Autodesk Inventor part; units mm, degrees
ref_plane "YZ Plane" through (0, 0, 0) normal (1, 0, 0) x (0, 1, 0)
ref_plane "XZ Plane" through (0, 0, 0) normal (0, 1, 0) x (-1, 0, 0)
ref_plane "XY Plane" through (0, 0, 0) normal (0, 0, 1) x (1, 0, 0)
sketch "Náčrt1" plane through (0, 0, 0) normal (1, 0, 0) x (0, 1, 0)
  line L0 (0, 0) -> (0, -50)
  line L1 (0, -50) -> (80, -50)
  line L2 (80, -50) -> (80, 0)
  line L3 (80, 0) -> (0, 0)
  dimension "d0" = 50
  dimension "d1" = 80
  dimension "d2" = 50
extrude "Vysunutí1" add sketch "Náčrt1" along normal blind 50
sketch "Náčrt2" plane through (50, 0, 0) normal (1, 0, 0) x (0, 0, -1)
  line L0 (0, 0) -> (20, 0)
  line L1 (0, 0) -> (50, 0)
  line L2 (20, 0) -> (20, 15)
  line L3 (20, 15) -> (0, 15)
  line L4 (0, 80) -> (0, 0)
  line L5 (0, 0) -> (0, 15)
  line L6 (0, 80) -> (10, 80)
  line L7 (50, 80) -> (0, 80)
  line L8 (10, 80) -> (10, 65)
  line L9 (10, 65) -> (0, 65)
  line L10 (0, 80) -> (0, 65)
  dimension "d5" = 20
  dimension "d6" = 15
  dimension "d7" = 10
  dimension "d8" = 15
extrude "Vysunutí2" cut sketch "Náčrt2" against normal blind 50
sketch "Náčrt3" plane through (50, 0, 0) normal (1, 0, 0) x (0, 0, -1)
  line L0 (20, 0) -> (50, 0)
  line L1 (50, 0) -> (30, 0)
  line L2 (30, 0) -> (30, 80)
  line L3 (50, 80) -> (10, 80)
  line L4 (10, 80) -> (10, 65)
  line L5 (30, 80) -> (10, 80)
  line L6 (10, 80) -> (10, 65)
  line L7 (10, 65) -> (0, 65)
  line L8 (10, 65) -> (0, 65)
  line L9 (0, 15) -> (20, 15)
  line L10 (0, 65) -> (0, 15)
  line L11 (0, 15) -> (20, 15)
  line L12 (20, 15) -> (20, 0)
  line L13 (20, 15) -> (20, 0)
  line L14 (20, 0) -> (30, 0)
  point P0 (0, 0)
  dimension "d11" = 20
extrude "Vysunutí3" cut sketch "Náčrt3" against normal blind 20
properties part number "Martin-Probst-26673_obrazek_1"
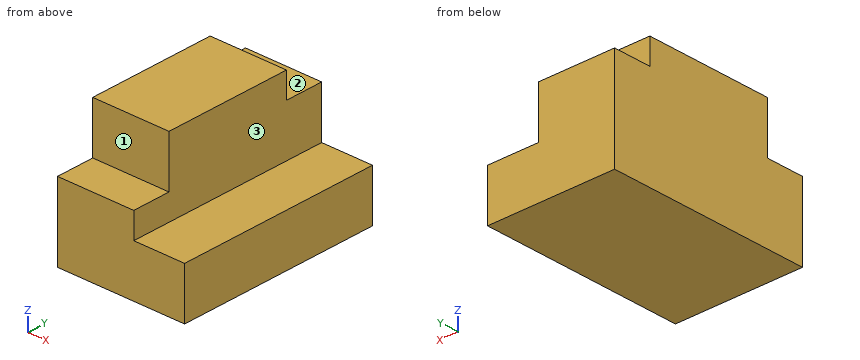
For this review, take the finished solid that the model builds, in its own axes (mm). Face numbers are marked on the shaded views. A direction names the side the tool comes from. Give positions to 0.01 mm unless a question says otherwise; leave off trailing zeros. Order: outer loops, then holes, each group sorted by start corner. A loop starts at its lowest first (then second) coordinate and runs counter-clockwise, first axis right, second up. Notation, with made-up numbers: (2.5, 15.5) - (57.5, 15.5) arc R18 ccw to (57.5, 38.5) - close; hole circle Ø10 at (20.25, 56). An arc over 180 degrees is marked (long way). Answer as a JSON object with one key per item and string values. Group by question number.
Item 1: Take a section at C-C on z = -28. Give the boundary of the cut face in (x, y).
Item 2: Take a section at B-B on x = 11.5. Give the boundary of the cut face in (y, z).
Item 3: Machinability: for the marked faces 1, 2 and 3, which of the approach directions +Z, -Z, +X, -X, +Y, -Y give a long, thin tool a straight path to every point of the face, cutting with its end or side? Answer none if there is none.
Item 4: Take a section at A-A on y = 52. Give the boundary of the cut face in (x, z), and give its area (3 significant figures).
Item 5: Clearance check with flat-ended pins moving along their axes: pin 1 Ø12 at (y, z) = (16, -19) entering from -X; pin 2 Ø4.5 at (x, y) = (17.5, 10) entering from +Z; pin 3 Ø10 at (x, y) = (37, 58.5) entering from +Z; pin 4 Ø10 at (x, z) = (11.5, -13) entering from -Y. State where each tip first meets the part, or that it passes through.
Item 6: Take a section at D-D on y = 14. Give the boundary of the cut face in (x, z).
Item 7: Wall thickness on line 1 along X through (y, z) = (39.5, -10); line 2 along Z through (x, y) = (35, 16); line 3 along Z through (x, y) = (21, 5): over which ranges is each line inside the solid? List them lowest first.
Reported:
{
 "1": {"outline": "(0, 0) - (30, 0) - (30, 80) - (0, 80) - close"},
 "2": {"outline": "(0, -50) - (80, -50) - (80, -10) - (65, -10) - (65, 0) - (15, 0) - (15, -20) - (0, -20) - close"},
 "3": {"face 1": "+Z, +X, -X, -Y", "face 2": "+Z, +X, -X, +Y", "face 3": "+Z, +X, +Y, -Y"},
 "4": {"outline": "(0, -50) - (50, -50) - (50, -30) - (30, -30) - (30, 0) - (0, 0) - close", "area": "1,900 mm^2"},
 "5": {"pin 1": "x = 0", "pin 2": "z = -20", "pin 3": "z = -30", "pin 4": "y = 15"},
 "6": {"outline": "(0, -50) - (50, -50) - (50, -30) - (30, -30) - (30, -20) - (0, -20) - close"},
 "7": {"line 1": "0 to 30", "line 2": "-50 to -30", "line 3": "-50 to -20"}
}
